Geometry: see drawing. Coordinates: mm, zero at the bounding-box minimum. A direction names the side the tool comes from. Give positions to 0.01 mm unless a question says otherwise; leave off trailing zeros. Write each loop counter-clockwise with the first axis right and the second up, starting at its lowest first coordinate (ties: lowest second). Pieces come first, ordered by that corner, then holes. Notation, with made-up numbers: M 32,-27.75 L 53,-27.75 A23 cw 53,-12.75 Z; hole C 55,84.25 d4. An arc over 180 degrees is marked long. Use a Markdown table: item, result. Add a question column.
(1) Material intervals for L1, parallel to X at y = 27, z = 27; L2, parallel to Y at x = 5, z = 46; L3, parallel to X at y = 3.5, z = 52, sorted ascending.
(2) Reachability of the marked faces 4, 5 and 6 from +Z, -Z, +X, -X, +Y, -Y: full face, straight path, thin tool, end or side. Return the list, or none.
(3) Pin query (flat end, axial travel): pin 1 Ø1 at (x, z) = (26, 54) entering from +Y; pin 2 Ø1.5 at (y, z) = (21, 51.5) entering from -X; pin 3 Ø8 at (x, y) = (35.5, 31) entering from +Z. Return the tip coordinate at first contact, or that it passes through.
(4) Cut plane B-B (y = 35). Output: boundary loops of the cut face in (x, z), plus the area to 3 significant figures.
(5) Draft query along X for the marked faces 1, 2 and 3. Return one class per face: released by +X, released by -X, zero draft, split by the parting line, or undercut.
(6) Cut plane C-C (z = 45). Output: boundary loops of the cut face in (x, y) (1 decimal), plus the area to 3 significant figures.
(7) Cut plane D-D (y = 20). Output: boundary loops of the cut face in (x, z).
(8) Cut plane A-A (x = 10.5). Output: boundary loops of the cut face in (y, z), plus the area to 4 significant figures.
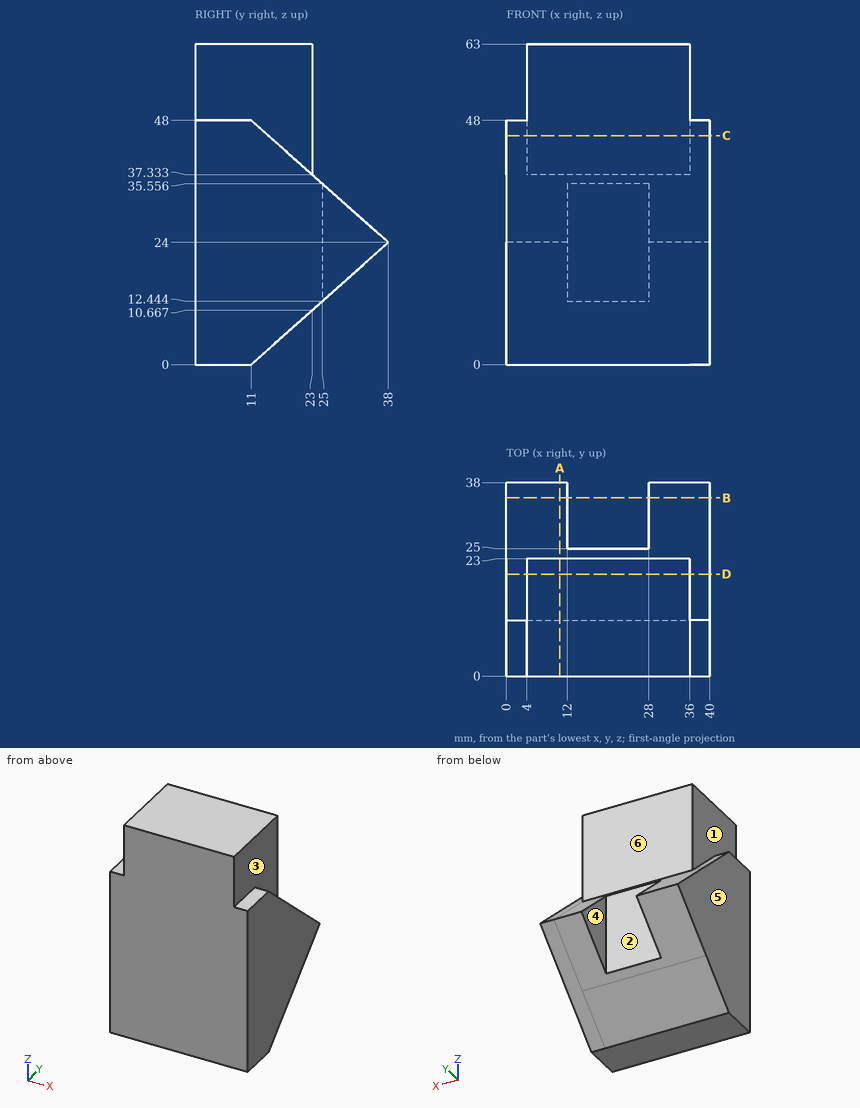
Answer list:
| question | item | result |
|---|---|---|
| 1 | L1 | 0 to 12, 28 to 40 |
| 1 | L2 | 0 to 23 |
| 1 | L3 | 4 to 36 |
| 2 | face 4 | +Z, -Z, +Y |
| 2 | face 5 | +Z, -Z, -X, +Y, -Y |
| 2 | face 6 | +Z, +X, -X, +Y |
| 3 | pin 1 | y = 23 |
| 3 | pin 2 | x = 4 |
| 3 | pin 3 | z = 33.78 |
| 4 | outline | M 0,21.33 L 12,21.33 L 12,26.67 L 0,26.67 Z; M 28,21.33 L 40,21.33 L 40,26.67 L 28,26.67 Z |
| 4 | area | 128 mm² |
| 5 | face 1 | released by -X |
| 5 | face 2 | undercut |
| 5 | face 3 | released by +X |
| 6 | outline | M 0,0 L 40,0 L 40,14.4 L 36,14.4 L 36,23 L 4,23 L 4,14.4 L 0,14.4 Z |
| 6 | area | 851 mm² |
| 7 | outline | M 0,8 L 40,8 L 40,40 L 36,40 L 36,63 L 4,63 L 4,40 L 0,40 Z |
| 8 | outline | M 0,0 L 11,0 L 38,24 L 23,37.33 L 23,63 L 0,63 Z |
| 8 | area | 1,585 mm² |
